```python
from build123d import *

# Parameters (mm, degrees)
SKETCH_1_R      = 2.05
SKETCH_1_R_2    = 11.5
SKETCH_1_R_3    = 1.5
SKETCH_1_R_4    = 9.525
SKETCH_1_W      = 2.1
SKETCH_1_H      = 8.1
EXTRUDE_1_DEPTH = 2
FILLET_2_R      = 3
FILLET_3_R      = 19
FILLET_4_R      = 14
FILLET_5_R      = 3


with BuildPart() as part:
    # 草图1 → 凸台-拉伸1 (new body)
    with BuildSketch(Plane.XY):
        with BuildLine():
            Line((-4.357142857, -0.045714286), (-4.357142857, 41.804285714))
            Line((-4.357142857, 41.804285714), (9.742857143, 41.804285714))
            Line((9.742857143, 41.804285714), (9.742857143, 14.954285714))
            Line((9.742857143, 14.954285714), (14.742857143, 14.954285714))
            Line((14.742857143, 14.954285714), (14.742857143, 41.804285714))
            Line((14.742857143, 41.804285714), (228.285977906, 41.804285714))
            Line((228.285977906, 41.804285714), (228.285977906, 65.804285714))
            Line((228.285977906, 65.804285714), (243.821285799, 65.804285714))
            Line((243.821285799, 65.804285714), (243.821285799, 41.804285714))
            Line((243.821285799, 41.804285714), (271.642857143, 30.954285714))
            ThreePointArc((271.642857143, 30.954285714), (302.642857143, -0.045714286), (271.642857143, -31.045714286))
            Line((271.642857143, -31.045714286), (240.642857143, -41.895714286))
            Line((240.642857143, -41.895714286), (-4.357142857, -41.895714286))
            Line((-4.357142857, -41.895714286), (-4.357142857, -0.045714286))
        make_face()
        with Locations((1.642857143, 29.954285714)):
            Circle(SKETCH_1_R, mode=Mode.SUBTRACT)
        with Locations((1.642857143, -0.045714286)):
            Circle(SKETCH_1_R, mode=Mode.SUBTRACT)
        with Locations((1.642857143, -30.045714286)):
            Circle(SKETCH_1_R, mode=Mode.SUBTRACT)
        with Locations((51.642857143, -0.045714286)):
            Circle(SKETCH_1_R_2, mode=Mode.SUBTRACT)
        with Locations((51.642857143, -14.045714286)):
            Circle(SKETCH_1_R_3, mode=Mode.SUBTRACT)
        with Locations((37.642857143, -0.045714286)):
            Circle(SKETCH_1_R_3, mode=Mode.SUBTRACT)
        with Locations((51.642857143, 13.954285714)):
            Circle(SKETCH_1_R_3, mode=Mode.SUBTRACT)
        with Locations((65.642857143, -0.045714286)):
            Circle(SKETCH_1_R_3, mode=Mode.SUBTRACT)
        with Locations((271.642857143, -0.045714286)):
            Circle(SKETCH_1_R_4, mode=Mode.SUBTRACT)
        with Locations((41.642857143, 35.954285714)):
            Circle(SKETCH_1_R, mode=Mode.SUBTRACT)
        with Locations((136.642857143, 35.954285714)):
            Circle(SKETCH_1_R, mode=Mode.SUBTRACT)
        with Locations((231.642857143, 35.954285714)):
            Circle(SKETCH_1_R, mode=Mode.SUBTRACT)
        with Locations((136.642857143, -36.045714286)):
            Circle(SKETCH_1_R, mode=Mode.SUBTRACT)
        with Locations((231.642857143, -36.045714286)):
            Circle(SKETCH_1_R, mode=Mode.SUBTRACT)
        with Locations((41.642857143, -36.045714286)):
            Circle(SKETCH_1_R, mode=Mode.SUBTRACT)
        with Locations((1.642857143, 14.954285714)):
            Rectangle(SKETCH_1_W, SKETCH_1_H, mode=Mode.SUBTRACT)
        with Locations((1.642857143, -15.045714286)):
            Rectangle(SKETCH_1_W, SKETCH_1_H, mode=Mode.SUBTRACT)
        with BuildLine():
            Line((139.521536799, -2.167034629), (111.571536799, 25.782965371))
            ThreePointArc((111.571536799, 25.782965371), (111.571536799, 30.025606058), (115.814177486, 30.025606058))
            Line((115.814177486, 30.025606058), (143.764177486, 2.075606058))
            ThreePointArc((143.764177486, 2.075606058), (143.764177486, -2.167034629), (139.521536799, -2.167034629))
        make_face(mode=Mode.SUBTRACT)
        Polygon((95.965816792, 27.904285714), (135.122522002, -11.252419496), (135.122522002, -27.867735073), (72.8281641, -27.867735073), (72.8281641, 27.904285714), align=None, mode=Mode.SUBTRACT)
        Polygon((9.742857143, -4.38924766), (30.529534128, -4.38924766), (41.642857143, -27.867735073), (9.742857143, -27.867735073), align=None, mode=Mode.SUBTRACT)
        Polygon((152.259089612, -26.603879462), (230.464406562, 25.782965371), (152.259089612, 25.782965371), align=None, mode=Mode.SUBTRACT)
        with BuildLine():
            Line((243.833851294, -2.236708437), (215.549580047, -30.520979685))
            ThreePointArc((215.549580047, -30.520979685), (211.167591744, -30.520979685), (211.167591744, -26.138991382))
            Line((211.167591744, -26.138991382), (239.451862991, 2.145279866))
            ThreePointArc((239.451862991, 2.145279866), (243.833851294, 2.145279866), (243.833851294, -2.236708437))
        make_face(mode=Mode.SUBTRACT)
    extrude(amount=EXTRUDE_1_DEPTH)

    # 圆角2
    fillet_2_edges = [part.edges().sort_by_distance(p)[0] for p in [
        (41.642857143, -27.867735073, 1),
        (30.529534128, -4.38924766, 1),
        (9.742857143, -4.38924766, 1),
        (9.742857143, -27.867735073, 1),
        (72.8281641, -27.867735073, 1),
        (135.122522002, -27.867735073, 1),
        (135.122522002, -11.252419496, 1),
        (95.965816792, 27.904285714, 1),
        (72.8281641, 27.904285714, 1),
        (152.259089612, -26.603879462, 1),
        (230.464406562, 25.782965371, 1),
        (152.259089612, 25.782965371, 1),
        (243.821285799, 65.804285714, 1),
    ]]
    fillet(fillet_2_edges, radius=FILLET_2_R)

    # 圆角3
    fillet_3_edges = [part.edges().sort_by_distance(p)[0] for p in [
        (14.742857143, 41.804285714, 1),
        (228.285977906, 41.804285714, 1),
        (243.821285799, 41.804285714, 1),
    ]]
    fillet(fillet_3_edges, radius=FILLET_3_R)

    # 圆角4
    fillet_4_edges = [part.edges().sort_by_distance(p)[0] for p in [
        (-4.357142857, -41.895714286, 1),
    ]]
    fillet(fillet_4_edges, radius=FILLET_4_R)

    # 圆角5
    fillet_5_edges = [part.edges().sort_by_distance(p)[0] for p in [
        (-4.357142857, 41.804285714, 1),
        (9.742857143, 41.804285714, 1),
    ]]
    fillet(fillet_5_edges, radius=FILLET_5_R)


solid = part.part
```
Part model, mm, in its own coordinate system. A direction names the side the tool comes from. Coordinates: 2 decimals unless noted, no trailing zeros. Order: outer loops, then holes, each group sorted by start corner. A loop starts at its lowest first (then second) coordinate and runs counter-clockwise, first axis right, second up. Notation, with made-up numbers: (48.25, 32) - (68.25, 32) arc R19 ccw to (68.25, 63) - close; hole circle Ø7 at (-8.75, 14.25). An arc over 180 degrees is marked (long way). Return JSON: item names as keys, results as strings. Group by question number.
Item 1: Cut at C-C (z = 1.1). State how many separate pieces and enclosed holes the cut face has, plus the area to 3 significant figures.
Item 2: Drill centre lines: probe 1 along X at (y, z) = (-16.5, 1.25); probe 2 along Y at (x, z) = (215, 0.6); probe 3 along X at (y, z) = (5.5, 0.2). Where is each one in solid material? Low to high. Write a range as from..to.
Item 3: Cut at B-B (x = 23). List the corners of the cut face in (y, z).
Item 4: Which spindle directions (+Z, -Z, +X, -X, +Y, -Y) get a long thin tool onto all of the face, cutting with end or side? Do faces 4 (the face through (247.045, 44.2, 1.014)), 5 (the face through (35.42, -14.72, 0.99)), 6 (the face through (20.46, 36.39, 1.01)). Say none if no direction does.
Item 5: Pull direction Y, two halves, no side cores. Call faces 1 (the face through (263.67, 34.063, 0.986)), 2 (the face through (302.635, 0.636, 0.986)), 3 (the face through (243.79, 2.19, 0.99)): pulls with the +Y half, pulls with the -Y half, needs draft (parallel to the pull), parting line crosses it, or undercut.
Item 6: Pin check, flat tips, straight feed: pin 1 (4.5 mm diameter, centred on x = 1.64, y = 29.95, fed in from -Z); pin 2 (0.6 mm diameter, centred on y = 6, z = 1, fed in from +X); pin 3 (1 mm diameter, centred on y = 60.5, z = 0.5, fed in from +X); pin 4 (0.6 mm diameter, centred on x = 1, z = 1, fed in from +Y). Stop position of each tip, or through.
Item 7: Cut at A-A (x = 80.5). List the corners of the cut face in (y, z).
Check values:
{
 "1": {"separate pieces": "1", "enclosed holes": "22", "area": "17,800 mm2"},
 "2": {"probe 1": "x = -4.36..0.59, 2.69..9.74, 36.26..72.83, 135.12..152.26, 167.34..220.81, 229.57..297.92", "probe 2": "y = -41.9..-30.96, -22.31..15.42, 25.78..42.68", "probe 3": "x = -4.36..41.57, 61.72..72.83, 118.37..131.85, 140.34..152.26, 200.19..263.9, 279.39..302.14"},
 "3": {"outline": "(-41.9, 0) - (-27.87, 0) - (-27.87, 2) - (-41.9, 2) - close; (-4.39, 0) - (38.48, 0) - (38.48, 2) - (-4.39, 2) - close"},
 "4": {"face 4": "+Z, -Z, +X, +Y", "face 5": "+Z, -Z", "face 6": "+Z, -Z, +Y"},
 "5": {"face 1": "pulls with the +Y half", "face 2": "parting line crosses it", "face 3": "undercut"},
 "6": {"pin 1": "stops at z = 0", "pin 2": "stops at x = 302.11", "pin 3": "stops at x = 243.82", "pin 4": "stops at y = 41.8"},
 "7": {"outline": "(-41.9, 0) - (-27.87, 0) - (-27.87, 2) - (-41.9, 2) - close; (27.9, 0) - (41.8, 0) - (41.8, 2) - (27.9, 2) - close"}
}
